Model file for the job. Use its own axes, mm. A direction names the side the tool comes from. Give positions to 0.01 mm unless a question says otherwise; leave off trailing zeros. Loops run counter-clockwise (first coordinate to the right, second up) from the corner with the lowest first, then second, coordinate; pieces in that order, holes last. Notation, with made-up numbers: M 68,-24 L 84,-24 A17 cw 84,-9 Z; hole C 63.25,85 d9. An arc over 180 degrees is marked long. Answer in a Markdown table with one row per item.
```python
from build123d import *

# Parameters (mm, degrees)
RESSALTO_EXTRUS_O1_DEPTH = 4.5


with BuildPart() as part:
    # Esboço1 → Ressalto-extrusão1 (new body, symmetric)
    with BuildSketch(Plane.XY):
        with BuildLine():
            ThreePointArc((90.369647409, -7.243523717), (97.877064824, -0.841102514), (92.047248027, 7.119145574))
            Line((92.047248027, 7.119145574), (4.614891567, 23.959607172))
            ThreePointArc((4.614891567, 23.959607172), (-5.96196459, 23.660409511), (-15.417653704, 18.911794052))
            Line((-15.417653704, 18.911794052), (-45.010991752, -5.213883118))
            ThreePointArc((-45.010991752, -5.213883118), (-47.432888855, -12.709604263), (-41.587603866, -17.990140644))
            Line((-41.587603866, -17.990140644), (-3.896182749, -24.086920932))
            ThreePointArc((-3.896182749, -24.086920932), (4.853764128, -23.912360272), (12.979282584, -20.661515521))
            Line((12.979282584, -20.661515521), (33.738260666, -7.621008284))
            ThreePointArc((33.738260666, -7.621008284), (38.064016153, -5.740396954), (42.753139424, -5.229532527))
            Line((42.753139424, -5.229532527), (90.369647409, -7.243523717))
        make_face()
        with BuildLine():
            ThreePointArc((-13.522040544, 16.586573471), (-5.228936157, 20.751342768), (4.047486866, 21.013753831))
            Line((4.047486866, 21.013753831), (91.479843326, 4.173292233))
            ThreePointArc((91.479843326, 4.173292233), (94.897322138, -0.493060095), (90.496422274, -4.246203558))
            Line((90.496422274, -4.246203558), (42.87991429, -2.232212369))
            ThreePointArc((42.87991429, -2.232212369), (37.294780203, -2.840694201), (32.142447233, -5.080658015))
            Line((32.142447233, -5.080658015), (11.383469151, -18.121165252))
            ThreePointArc((11.383469151, -18.121165252), (4.25698985, -20.972315976), (-3.417143886, -21.12541426))
            Line((-3.417143886, -21.12541426), (-41.108565003, -15.028633972))
            ThreePointArc((-41.108565003, -15.028633972), (-44.535111376, -11.933147128), (-43.115378592, -7.539103698))
            Line((-43.115378592, -7.539103698), (-13.522040544, 16.586573471))
        make_face(mode=Mode.SUBTRACT)
    extrude(amount=RESSALTO_EXTRUS_O1_DEPTH, both=True)


solid = part.part
```
Q1. Saw through at B-B (x = -25). Give the cut face in (y, z).
Reported:
| item | result |
|---|---|
| outline | M -20.67,-4.5 L -17.63,-4.5 L -17.63,4.5 L -20.67,4.5 Z; M 7.23,-4.5 L 11.1,-4.5 L 11.1,4.5 L 7.23,4.5 Z |
Q2. Probe probe 1 along Y at (x, z) = (0, 1.75); probe 2 along Y at (x, z) = (-16, -3.5); probe 3 along X at (y, z) = (-9.5, 2). List the from-to ranges inside material, lowest first.
Reported:
| item | result |
|---|---|
| probe 1 | -24.4 to -21.4, 21.4 to 24.4 |
| probe 2 | -22.13 to -19.09, 14.57 to 18.44 |
| probe 3 | -47.56 to -44.47, 25.11 to 30.75 |
Q3. Saw through at A-A (z = -0.25). Give the cut face in (x, y), and give its area (3 significant figures).
Reported:
| item | result |
|---|---|
| outline | M -45.01,-5.21 A7.25 ccw -41.59,-17.99 L -3.9,-24.09 A24.4 ccw 12.98,-20.66 L 33.74,-7.62 A15.7 cw 42.75,-5.23 L 90.37,-7.24 A7.25 ccw 92.05,7.12 L 4.61,23.96 A24.4 ccw -15.42,18.91 Z; hole M -43.12,-7.54 A4.25 ccw -41.11,-15.03 L -3.42,-21.13 A21.4 ccw 11.38,-18.12 L 32.14,-5.08 A18.7 cw 42.88,-2.23 L 90.5,-4.25 A4.25 ccw 91.48,4.17 L 4.05,21.01 A21.4 ccw -13.52,16.59 Z |
| area | 945 mm² |
Q4. Saw through at C-C (y = 15). Give the cut face in (x, z), and give its area (3 significant figures).
Reported:
| item | result |
|---|---|
| outline | M -20.22,-4.5 L -15.47,-4.5 L -15.47,4.5 L -20.22,4.5 Z; M 35.27,-4.5 L 51.13,-4.5 L 51.13,4.5 L 35.27,4.5 Z |
| area | 185 mm² |
Q5. Drop flat-ended pins along their axis: pin 1 (8 mm diameter, centred on x = 43.5, y = -6, fed in from +Z); pin 2 (4 mm diameter, centred on x = 45.5, y = -7.5, fed in from +Z). Give the stop position or say it passes through.
Reported:
| item | result |
|---|---|
| pin 1 | z = 4.5 |
| pin 2 | through |
Q6. 3-axis set-ups, long thin cutter, end or side, ignore diameter. For faces 1 (the face through (-22, -18.12, 0.06)), 2 (the face through (23.213, -14.233, 0.063)), 3 (the face through (66.228, -6.222, 0.063)): which of +Z, -Z, +X, -X, +Y, -Y reach the whole face in a straight line?
Reported:
| item | result |
|---|---|
| face 1 | +Z, -Z |
| face 2 | +Z, -Z, +X, -Y |
| face 3 | +Z, -Z, -Y |
